from build123d import *

# Parameters (mm, degrees)
F0_W      = 113
F0_H      = 26
F1_DEPTH  = 64
F2_W      = 25
F2_H      = 36.5019804899
F3_DEPTH  = 50.8
F4_W      = 25
F4_H      = 65.5092679775
F5_DEPTH  = 50.8
F6_DEPTH  = 25.4
F7_W      = 25
F7_H      = 54.8469666392
F8_DEPTH  = 50.8
F9_W      = 35
F9_H      = 17
F10_DEPTH = 50.8
F11_SIZE  = 10
F12_SIZE  = 10


# Not quite as in the source:
# - a feature of the source that left no trace in its solid (it failed there, or was rolled back) is left out


with BuildPart() as f1:
    # F0 (on Top) → F1 (new body)
    with BuildSketch(Plane.XY):
        with Locations((5.4938797247, 11.7718060501)):
            Rectangle(F0_W, F0_H)
    extrude(amount=F1_DEPTH)

    # F2 (on Front) → F3 (cut, symmetric)
    with BuildSketch(Plane.XZ):
        with Locations((5.4938797247, 48.2509902449)):
            Rectangle(F2_W, F2_H)
    extrude(amount=F3_DEPTH, both=True, mode=Mode.SUBTRACT)

    # F4 (on Front) → F5 (cut, symmetric)
    with BuildSketch(Plane.XZ):
        with Locations((-38.5061202753, 45.7546339888)):
            Rectangle(F4_W, F4_H)
    extrude(amount=F5_DEPTH, both=True, mode=Mode.SUBTRACT)

    # F6 (add): faces of the model
    f6_faces = [f1.faces().sort_by_distance(p)[0] for p in [
        (16.4788023799, -1.2281939499, 27.8806540043),
        (16.4788023799, 24.7718060501, 27.8806540043),
    ]]
    extrude(f6_faces, amount=F6_DEPTH, dir=(0, -1, 0))

    # F7 (on Front) → F8 (cut, symmetric)
    with BuildSketch(Plane.XZ):
        with Locations((49.4938797247, 40.4234833196)):
            Rectangle(F7_W, F7_H)
    extrude(amount=F8_DEPTH, both=True, mode=Mode.SUBTRACT)

    # F9 (on Front) → F10 (cut, symmetric)
    with BuildSketch(Plane.XZ):
        with Locations((5.4938797247, 8.5)):
            Rectangle(F9_W, F9_H)
    extrude(amount=F10_DEPTH, both=True, mode=Mode.SUBTRACT)

    # F11
    f11_edges = [f1.edges().sort_by_distance(p)[0] for p in [
        (61.99388, -26.628194, 6.5),
    ]]
    chamfer(f11_edges, length=F11_SIZE)

    # F12
    f12_edges = [f1.edges().sort_by_distance(p)[0] for p in [
        (-51.00612, -26.628194, 6.5),
    ]]
    chamfer(f12_edges, length=F12_SIZE)


solid = f1.part
Verification items for the finished model (mm, model axes). A direction names the side the tool comes from. Give positions to 0.01 mm unless a question says otherwise; leave off trailing zeros. Order: outer loops, then holes, each group sorted by start corner. A loop starts at its lowest first (then second) coordinate and runs counter-clockwise, first axis right, second up. Notation, with made-up numbers: M 73.5,68.5 L 131.5,68.5 A20 ccw 131.5,107.5 Z; hole C 0,28 d5. An arc over 180 degrees is marked long. Answer as a JSON object with one key per item and string values. Group by question number.
1) Depth check by flat-ended pin: pin 1 Ø5 at (y, z) = (-13.5, 23) entering from +X; pin 2 Ø6 at (y, z) = (-20.5, 11.5) entering from +X; pin 3 Ø10 at (y, z) = (6, 24.5) entering from -X. Enter the tip coordinate at first touch or a pass-through.
2) Scan lines: line 1 along X through (y, z) = (-13, 39); line 2 along X through (y, z) = (15, 9); line 3 along X through (y, z) = (10, 18). Record each from-to range of solid material in increasing order. Write a range as [from, to].
3) Cross-section at C-C (y = 14). Enter the section's corners in (x, z).
4) Cross-section at A-A (z = 35.5). Enter the section's corners in (x, y).
5) Cross-section at D-D (x = -38). Enter the section's corners in (y, z), then the cut area to 3 significant figures.
6) Access from +Z, -Z, +X, -X, +Y, -Y to the whole of each face (thin tool, end or side, straight path). Record for faces 1 (the face through (17.994, -1, 47)), 2 (the face through (5, -1, 17)), 3 (the face through (49, -1, 13)).
7) Cross-section at B-B (z = 11.5). Enter the section's corners in (x, y).
Result sheet:
{
 "1": {"pin 1": "stops at x = 36.99", "pin 2": "stops at x = 61.12", "pin 3": "stops at x = -26.01"},
 "2": {"line 1": "x = [-26.01, -7.01], [17.99, 36.99]", "line 2": "x = [-51.01, -12.01], [22.99, 61.99]", "line 3": "x = [-26.01, 36.99]"},
 "3": {"outline": "M -51.01,0 L -12.01,0 L -12.01,17 L 22.99,17 L 22.99,0 L 61.99,0 L 61.99,13 L 36.99,13 L 36.99,64 L 17.99,64 L 17.99,30 L -7.01,30 L -7.01,64 L -26.01,64 L -26.01,13 L -51.01,13 Z"},
 "4": {"outline": "M -26.01,-26.63 L -7.01,-26.63 L -7.01,24.77 L -26.01,24.77 Z; M 17.99,-26.63 L 36.99,-26.63 L 36.99,24.77 L 17.99,24.77 Z"},
 "5": {"outline": "M -26.63,0 L 24.77,0 L 24.77,13 L -26.63,13 Z", "area": "668 mm2"},
 "6": {"face 1": "+Z, +Y, -Y", "face 2": "-Z, +Y, -Y", "face 3": "+Z, +X, +Y, -Y"},
 "7": {"outline": "M -51.01,-16.63 L -41.01,-26.63 L -12.01,-26.63 L -12.01,24.77 L -51.01,24.77 Z; M 22.99,-26.63 L 51.99,-26.63 L 61.99,-16.63 L 61.99,24.77 L 22.99,24.77 Z"}
}
